Model file for the job. Use its own axes, mm. A direction names the side the tool comes from. Give positions to 0.01 mm unless a question says otherwise; leave off trailing zeros. Order: outer loops, then holes, each group sorted by start corner. A loop starts at its lowest first (then second) coordinate and runs counter-clockwise, first axis right, second up. Notation, with made-up numbers: M 2.5,31.5 L 49.5,31.5 A18 cw 49.5,56.5 Z; hole C 24.5,47 d6. An arc over 180 degrees is marked long. Return JSON: item names as keys, results as strings. Group by question number.
1. Slice it at A-A on x = 0. List the corners of the cut face in (y, z), then the cut area to 3 significant figures.
2. Pin check, flat tips, straight feed: pin 1 (8 mm diameter, centred on x = -11, z = 4, fed in from -Y); pin 2 (10 mm diameter, centred on y = -6, z = 16, fed in from +X); pin 3 (1 mm diameter, centred on x = 10.5, z = 5.5, fed in from -Y). Stop position of each tip, or through.
3. Two-plate mould, pull along X, no slides. Class faces 1 (the face through (7.13, 7.01, 12.49)), 2 (the face through (-4, 7, 13)), 3 (the face through (-7.997, 0.631, 6.591)): released by +X, released by -X, zero draft, split by the parting line, or undercut.
4. Slice it at C-C on z = 8.25. List the corners of the cut face in (x, y), then the cut area to 3 significant figures.
5. 3-axis set-ups, long thin cutter, end or side, ignore diameter. For faces 4 (the face through (-7.13, -7.01, 12.49)), 5 (the face through (7.01, -7.13, 12.49)), 6 (the face through (10, -3, 12)), 7 (the face through (-7.01, 7.13, 12.49)): which of +Z, -Z, +X, -X, +Y, -Y reach the whole face in a straight line?
6. Slice it at D-D on y = -11. List the corners of the cut face in (x, z), then the cut area to 3 significant figures.
7. Wall check: probe 1 along Y at (x, z) = (0, 7.75); probe 2 along X at (y, z) = (1.5, 9.75); probe 3 along Z at (x, y) = (-11.75, 9). Give the ranges that are in metal, low to high. Write a range as [from, to].
from build123d import *

# Parameters (mm, degrees)
SKETCH_1_R      = 15
EXTRUDE_1_DEPTH = 12
SKETCH_2_R      = 10
EXTRUDE_2_DEPTH = 1
SKETCH_3_R      = 7.5
EXTRUDE_3_DEPTH = 11
M5X0_81_D       = 4.2
M3X0_51_D       = 2.5


with BuildPart() as part:
    # Эскиз1 → Бобышка-Вытянуть1 (new body)
    with BuildSketch(Plane.XY):
        Circle(SKETCH_1_R)
    extrude(amount=EXTRUDE_1_DEPTH)

    # Эскиз2 → Бобышка-Вытянуть2 (add)
    with BuildSketch(Plane.XY.offset(12)):
        Circle(SKETCH_2_R)
    extrude(amount=EXTRUDE_2_DEPTH)

    # Эскиз3 → Бобышка-Вытянуть3 (add)
    with BuildSketch(Plane.XY.offset(13)):
        Circle(SKETCH_3_R)
    extrude(amount=EXTRUDE_3_DEPTH)

    # Отверстие обработанное метчиком M5x0.81 (through all)
    with Locations(Plane(origin=(0, 0, 0), x_dir=(-1, 0, 0), z_dir=(0, 0, -1))):
        with Locations((0, 10), (10, 0), (-10, 0), (0, -10)):
            Hole(M5X0_81_D / 2)

    # Отверстие обработанное метчиком M3x0.51 (through all)
    with Locations(Plane.XY.offset(24)):
        with Locations((-2.828427125, -2.828427125), (2.828427125, 2.828427125)):
            Hole(M3X0_51_D / 2)


solid = part.part
Result:
{
 "1": {"outline": "M -15,0 L -12.1,0 L -12.1,12 L -15,12 Z; M -7.9,0 L 7.9,0 L 7.9,13 L 7.5,13 L 7.5,24 L -7.5,24 L -7.5,13 L -7.9,13 Z; M 12.1,0 L 15,0 L 15,12 L 12.1,12 Z", "area": "440 mm2"},
 "2": {"pin 1": "stops at y = -13.27", "pin 2": "stops at x = 14.7", "pin 3": "stops at y = -11.18"},
 "3": {"face 1": "released by +X", "face 2": "zero draft", "face 3": "undercut"},
 "4": {"outline": "C 0,0 d30; hole C -10,0 d4.2; hole C -2.83,-2.83 d2.5; hole C 0,-10 d4.2; hole C 0,10 d4.2; hole C 2.83,2.83 d2.5; hole C 10,0 d4.2", "area": "642 mm2"},
 "5": {"face 4": "+Z, -X, -Y", "face 5": "+Z, +X, -Y", "face 6": "+Z", "face 7": "+Z, -X, +Y"},
 "6": {"outline": "M -10.2,0 L -1.85,0 L -1.85,12 L -10.2,12 Z; M 1.85,0 L 10.2,0 L 10.2,12 L 1.85,12 Z", "area": "200 mm2"},
 "7": {"probe 1": "y = [-15, -12.1], [-7.9, 7.9], [12.1, 15]", "probe 2": "x = [-14.92, -11.47], [-8.53, 8.53], [11.47, 14.92]", "probe 3": "z = [0, 12]"}
}
